Check sheet for the modelled part. Datum: model origin and axes. Units: mm. Face numbers are marked on the shaded views. A direction names the side the tool comes from. Coordinates: 2 decimals unless noted, no trailing zeros. Loops run counter-clockwise (first coordinate to the right, second up) from the corner with the lowest first, then second, coordinate; pieces in that order, holes last. Notation, with made-up numbers: (-38.75, -35) -> (-9.75, -35) arc R24 cw to (-9.75, -20) -> close; hole circle Ø8 at (-30, 2). An arc over 180 degrees is marked (long way). Use CSV: the item, a comma, the result in double quotes. Start each with the question number.
1. Sectioned sample at D-D, the plane z = 5.75. Record the cut outline in (x, y).
2. Gauge pin test, flat ends, axial feed: pin 1 (5 mm diameter, centred on x = 0.5, z = 6.5, fed in from -Y); pin 2 (1 mm diameter, centred on y = 57, z = -2.5, fed in from +X); pin 3 (3 mm diameter, centred on y = 24, z = 4.5, fed in from -X); pin 4 (2 mm diameter, centred on y = 11, z = 5, fed in from -X). Record the tip position at first contact, or that the pin passes through.
3. Thickness scan on L1, parallel to Y at x = 0, z = -8.25; L2, parallel to Y at x = -3.25, z = 0.25; L3, parallel to X at y = -1, z = 1. Record the ranges inside material, lowest first.
4. Sectioned sample at A-A, the plane z = 0. Record the cut outline in (x, y) (3 decimals), and give its area (3 significant figures).
5. Set-up check for the marked faces 1 and 2: record each of +Z, -Z, +X, -X, +Y, -Y from which the full face is reachable in a straight line by a thin tool's end or side.
6. Sectioned sample at C-C, the plane y = 22.5. Record the cut outline in (x, z) (3 decimals).
7. Sectioned sample at B-B, the plane x = 0. Record the cut outline in (y, z) (3 decimals), and give its area (3 significant figures).
```python
from build123d import *

# Parameters (mm, degrees)
SKETCH1_R           = 3.325
BOSS_EXTRUDE1_DEPTH = 69.2
SKETCH2_R           = 3.59
BOSS_EXTRUDE2_DEPTH = 6.82
BOSS_EXTRUDE3_DEPTH = 1.76


with BuildPart() as part:
    # Sketch1 → Boss-Extrude1 (new body)
    with BuildSketch(Plane(origin=(0, 0, 0), x_dir=(1, 0, 0), z_dir=(0, 1, 0))):
        Circle(SKETCH1_R)
    extrude(amount=BOSS_EXTRUDE1_DEPTH)

    # Sketch2 → Boss-Extrude2 (add)
    with BuildSketch(Plane(origin=(0, 69.2, 0), x_dir=(1, 0, 0), z_dir=(0, 1, 0))):
        Circle(SKETCH2_R)
    extrude(amount=BOSS_EXTRUDE2_DEPTH)

    # Sketch3 → Boss-Extrude3 (add)
    with BuildSketch(Plane(origin=(0, 76.02, 0), x_dir=(1, 0, 0), z_dir=(0, 1, 0))):
        with BuildLine():
            Line((-4.91772543, 1.370037078), (-2.65, 9.51))
            Line((-2.65, 9.51), (2.65, 9.51))
            Line((2.65, 9.51), (4.91772543, 1.370037078))
            ThreePointArc((4.91772543, 1.370037078), (5.105, 0), (4.91772543, -1.370037078))
            Line((4.91772543, -1.370037078), (2.65, -9.51))
            Line((2.65, -9.51), (-2.65, -9.51))
            Line((-2.65, -9.51), (-4.91772543, -1.370037078))
            ThreePointArc((-4.91772543, -1.370037078), (-5.105, 0), (-4.91772543, 1.370037078))
        make_face()
    extrude(amount=BOSS_EXTRUDE3_DEPTH)

    # Sketch4 → Revolve1 (revolve)
    with BuildSketch(Plane(origin=(0, 0, 0), x_dir=(0, 0, -1), z_dir=(1, 0, 0))):
        with BuildLine():
            Line((0, 0), (0, -9.35))
            Line((0, -9.35), (2, -9.35))
            Line((2, -9.35), (2.21, -1.3))
            ThreePointArc((2.21, -1.3), (2.536524, -0.451893662), (3.325, 0))
            Line((3.325, 0), (0, 0))
        make_face()
    revolve(axis=Axis((0, 0, 0), (0, -1, 0)))


solid = part.part
```
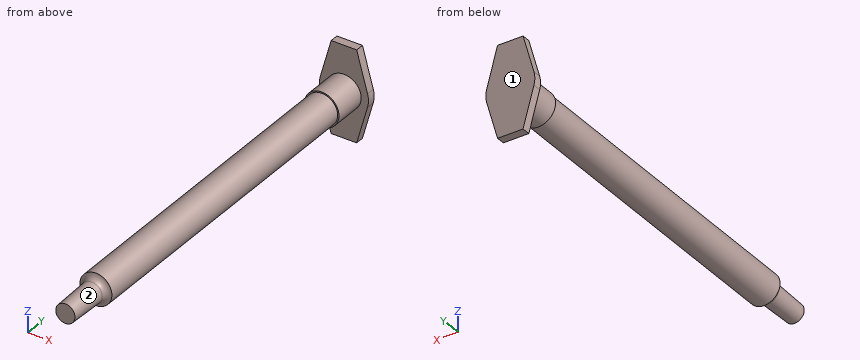
Completed:
1,outline,"(-3.7, 76.02) -> (3.7, 76.02) -> (3.7, 77.78) -> (-3.7, 77.78) -> close"
2,pin 1,"y = 76.02"
2,pin 2,"x = 2.66"
2,pin 3,"x = -1.43"
2,pin 4,"through"
3,L1,"76.02 to 77.78"
3,L2,"-0.01 to 77.78"
3,L3,"-2.02 to 2.02"
4,outline,"(-5.105, 76.02) -> (-3.59, 76.02) -> (-3.59, 69.2) -> (-3.325, 69.2) -> (-3.325, 0) arc R1.357 cw to (-2.21, -1.3) -> (-2, -9.35) -> (2, -9.35) -> (2.21, -1.3) arc R1.357 cw to (3.325, 0) -> (3.325, 69.2) -> (3.59, 69.2) -> (3.59, 76.02) -> (5.105, 76.02) -> (5.105, 77.78) -> (-5.105, 77.78) -> close"
4,area,"567 mm²"
5,face 1,"+Z, -Z, +X, -X, +Y"
5,face 2,"-Y"
6,outline,"circle Ø6.65 at (0, 0)"
7,outline,"(-9.35, -2) -> (-1.3, -2.21) arc R1.357 cw to (0, -3.325) -> (69.2, -3.325) -> (69.2, -3.59) -> (76.02, -3.59) -> (76.02, -9.51) -> (77.78, -9.51) -> (77.78, 9.51) -> (76.02, 9.51) -> (76.02, 3.59) -> (69.2, 3.59) -> (69.2, 3.325) -> (0, 3.325) arc R1.357 cw to (-1.3, 2.21) -> (-9.35, 2) -> close"
7,area,"583 mm²"
